The figure shows three views and two pictorial views of one solid part (mm, origin at its lowest corner). Answer the questions. A direction names the side the tool comes from. Round coordinates to 2 decimals unless told otherwise and drop trailing zeros. Order: outer loops, then holes, each group sorted by start corner. A loop starts at its lowest first (then second) coordinate and runs counter-clockwise, first axis right, second up. Notation, with made-up numbers: (-21, 17.25) - (10, 17.25) arc R22 cw to (10, 25.25) - close; hole circle Ø11 at (-21, 71). An arc over 180 degrees is marked (long way). Use CSV: the item, a comma, the result in double quotes.
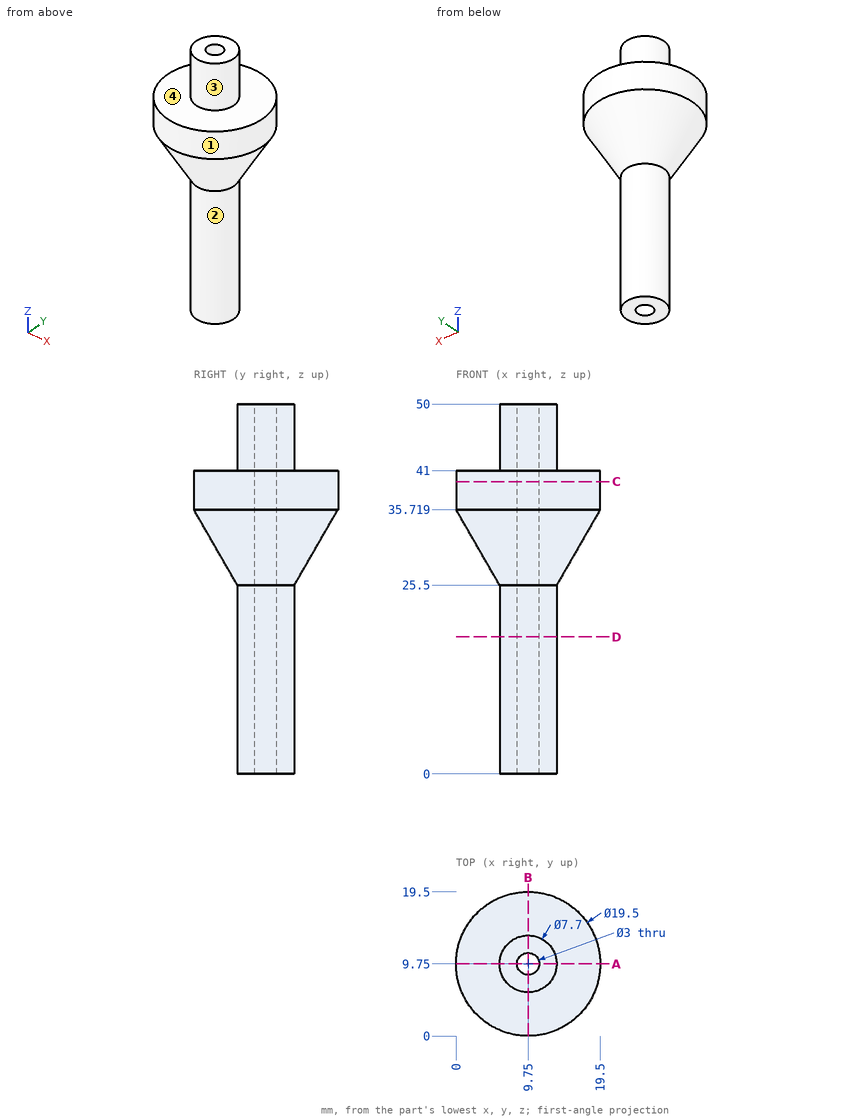
(1) Find section A-A (y = 9.75). Determine the outline of the cut face in (x, z).
Findings below:
outline,"(0, 35.72) - (5.9, 25.5) - (5.9, 0) - (8.25, 0) - (8.25, 50) - (5.9, 50) - (5.9, 41) - (0, 41) - close; (11.25, 0) - (13.6, 0) - (13.6, 25.5) - (19.5, 35.72) - (19.5, 41) - (13.6, 41) - (13.6, 50) - (11.25, 50) - close"
(2) Find the intervals of material crossed by L1, parallel to X at y = 9.75, z = 19.5; L2, parallel to X at y = 9.75, z = 39.5, in increasing order. Write a range as from..to.
Findings below:
L1,"x = 5.9..8.25, 11.25..13.6"
L2,"x = 0..8.25, 11.25..19.5"
(3) Find section C-C (z = 39.5). Determine the outline of the cut face in (x, y), and give its area (3 significant figures).
Findings below:
outline,"circle Ø19.5 at (9.75, 9.75); hole circle Ø3 at (9.75, 9.75)"
area,"292 mm²"
(4) For the marked faces 1 and 2, determine the directions among +Z, -Z, +X, -X, +Y, -Y from which every point of the face is accessible in a straight line to the end or side of a thin tool.
Findings below:
face 1,"+Z, -Z"
face 2,"-Z"
(5) Each of these flat-tipped pins is pushed along its axis until it touches: pin 1 (10 mm diameter, centred on y = 3.5, z = 36.5, fed in from +X); pin 2 (10 mm diameter, centred on x = 12, z = 41.5, fed in from -Y); pin 3 (6 mm diameter, centred on x = 16, z = 21, fed in from -Y); pin 4 (1.5 mm diameter, centred on x = 8.5, z = 12.5, fed in from -Y). Where does it stop, or does it pass through?
Findings below:
pin 1,"stops at x = 19.42"
pin 2,"stops at y = 0"
pin 3,"stops at y = 7.69"
pin 4,"stops at y = 5.93"
(6) The mould has two halves that part along X. Classify the marked faces 3 and 4: released by +X, released by -X, zero draft, split by the parting line, or undercut.
Findings below:
face 3,"split by the parting line"
face 4,"zero draft"
(7) Find section D-D (z = 18.5). Determine the outline of the cut face in (x, y), and give its area (3 significant figures).
Findings below:
outline,"circle Ø7.7 at (9.75, 9.75); hole circle Ø3 at (9.75, 9.75)"
area,"39.5 mm²"
